Verification items for this drawing (mm, ordinates from the low corner). A direction names the side the tool comes from. Coordinates: 2 decimals unless noted, no trailing zeros. Write each loop counter-clockwise with the first axis right and the second up, starting at its lowest first coordinate (ties: lowest second). Pieces come first, ordered by that corner, then holes. Notation, with made-up numbers: M -30.75,23 L 5.25,23 A25 cw 5.25,41 Z; hole C 82.25,58.5 d4. An arc over 180 degrees is marked long. Write each question's results on one line, items separated by ' | '.
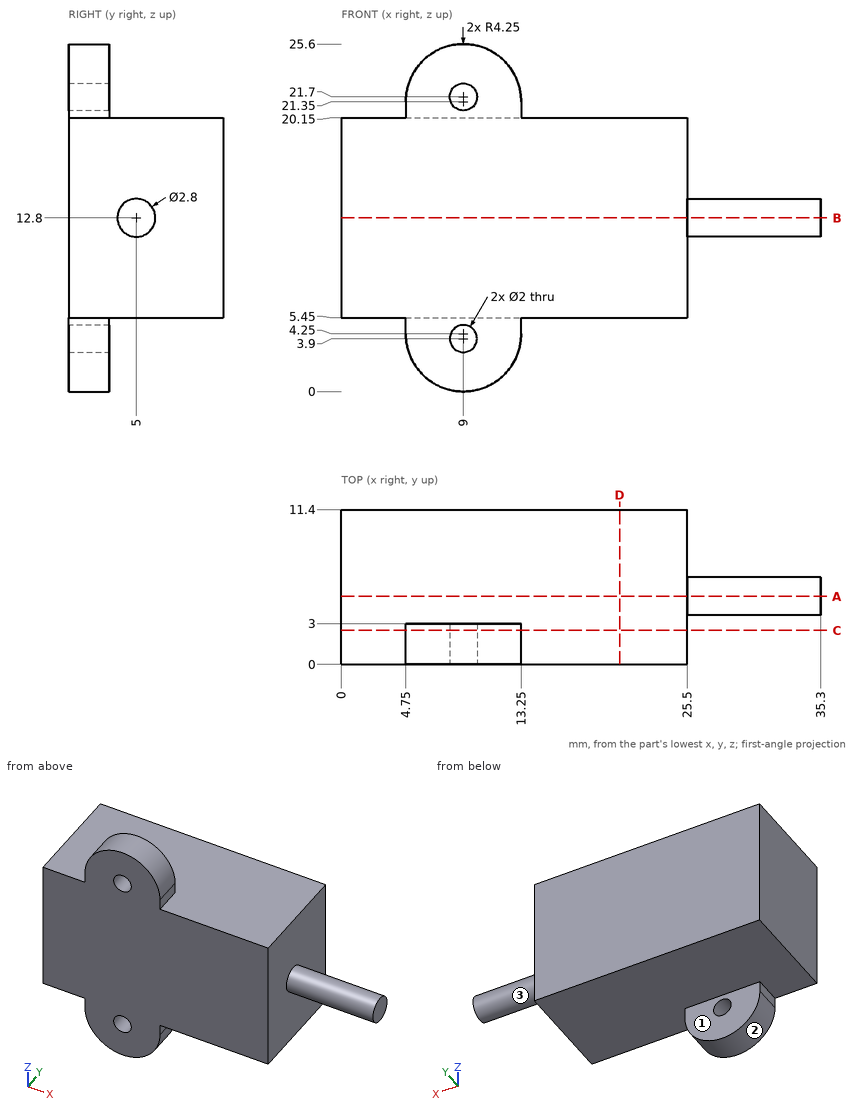
Q1. Sectioned sample at A-A on y = 5. Record the cut outline in (x, z), and give its area (3 significant figures).
Geometry check:
outline: M 0,5.45 L 25.5,5.45 L 25.5,11.4 L 35.3,11.4 L 35.3,14.2 L 25.5,14.2 L 25.5,20.15 L 0,20.15 Z | area: 402 mm2
Q2. Scan lines: probe 1 along Z at (x, y) = (5, 8.75); probe 2 along X at (y, z) = (2.25, 10.25); probe 3 along Y at (x, z) = (10.5, 23.5). Record each from-to range of solid material in increasing order.
Geometry check:
probe 1: z = 5.45 to 20.15 | probe 2: x = 0 to 25.5 | probe 3: y = 0 to 3
Q3. Sectioned sample at C-C on y = 2.5. Record the cut outline in (x, z).
Geometry check:
outline: M 0,5.45 L 4.75,5.45 L 4.75,4.25 A4.25 ccw 13.25,4.25 L 13.25,5.45 L 25.5,5.45 L 25.5,20.15 L 13.25,20.15 L 13.25,21.35 A4.25 ccw 4.75,21.35 L 4.75,20.15 L 0,20.15 Z; hole C 9,3.9 d2; hole C 9,21.7 d2
Q4. Depth check by flat-ended pin: P1, Ø4.5, axis at x = 11, z = 2, coming from the +Y side; P2, Ø1, axis at y = 1.5, z = 21, coming from the -X side; P3, Ø2, axis at x = 20.5, y = 9, coming from the +Z side. Enter the tip coordinate at first touch or a pass-through.
Geometry check:
P1: stops at y = 3 | P2: stops at x = 4.75 | P3: stops at z = 20.15
Q5. Access from +Z, -Z, +X, -X, +Y, -Y to the whole of each face (thin tool, end or side, straight path). Record for the marked faces 1, 2 and 3.
Geometry check:
face 1: -Z, +X, -X, +Y | face 2: -Z, +Y, -Y | face 3: +X
Q6. Sectioned sample at D-D on x = 20.5. Record the cut outline in (y, z), and give its area (3 significant figures).
Geometry check:
outline: M 0,5.45 L 11.4,5.45 L 11.4,20.15 L 0,20.15 Z | area: 168 mm2
Q7. Sectioned sample at B-B on z = 12.8. Record the cut outline in (x, y).
Geometry check:
outline: M 0,0 L 25.5,0 L 25.5,3.6 L 35.3,3.6 L 35.3,6.4 L 25.5,6.4 L 25.5,11.4 L 0,11.4 Z
